```python
from build123d import *

# Parameters (mm, degrees)
F0_W        = 31.6318599507
F0_H        = 42.7960464731
F0_W_2      = 4.3416279368
F0_H_2      = 18.813719973
F0_W_3      = 4.5483717695
F0_H_3      = 19.0204642713
F1_DEPTH    = 3.302
F3_DEPTH    = 0.254
F4_DEPTH    = 12.192
F5_DEPTH    = 7.62
F6_DEPTH    = 7.366
F7_R        = 5.08
F8_T1_DEPTH = 55.4253023246
F9_W        = 5.16293291
F9_H        = 4.0333122015
F9_W_2      = 5.5523253977
F9_H_2      = 4.3130330741
F9_H_3      = 3.302
F9_W_3      = 5.3753489628
F10_DEPTH   = 25.4
F11_R       = 2.4528409794
F12_R       = 1.2264204897


# Not quite as in the source:
# - a fillet or chamfer that OpenCascade refuses, or shapes differently, is made with other operations: its cross-section is extruded or revolved along the edge and cut away or added


with BuildPart() as f1:
    # F0 (on Front) → F1 (new body)
    with BuildSketch(Plane.XZ):
        with Locations((-0.3101159818, 8.9933718555)):
            Rectangle(F0_W, F0_H)
        with Locations((-6.3056976069, 9.4068599865)):
            Rectangle(F0_W_2, F0_H_2, mode=Mode.SUBTRACT)
        with Locations((5.5820937268, 9.5102321357)):
            Rectangle(F0_W_3, F0_H_3, mode=Mode.SUBTRACT)
    extrude(amount=F1_DEPTH)

    # F3 (add): a face of the model
    f3_faces = [f1.faces().sort_by_distance(p)[0] for p in [
        (-0.3101159818, -1.651, 30.391395092),
    ]]
    extrude(f3_faces, amount=F3_DEPTH)

    # F2 (on Top) → F4 (join)
    with BuildSketch(Plane.XY):
        with BuildLine():
            Line((-16.1260459572, -3.0640123878), (-16.1260459572, -5.3753489628))
            Line((-16.1260459572, -5.3753489628), (-16.1260459572, -23.9823255688))
            add(Edge.make_bspline(
                [(-16.1260459572, -23.9823255688), (-10.712885637, -26.1710511495), (-0.0173269949, -30.4956307693), (10.2353861269, -26.1356592233), (15.2990687639, -23.9823255688)],
                knots=[0, 0, 0, 0, 0.5061129111, 1, 1, 1, 1], degree=3))
            Line((15.2990687639, -23.9823255688), (15.2990687639, -5.1686046645))
            Line((15.2990687639, -5.1686046645), (15.2990687639, -3.0640123878))
            Line((15.2990687639, -3.0640123878), (-16.1260459572, -3.0640123878))
        make_face()
    extrude(amount=-F4_DEPTH)

    # F5 (add): a face of the model
    f5_faces = [f1.faces().sort_by_distance(p)[0] for p in [
        (-0.3946759913, -14.5235842944, 0),
    ]]
    extrude(f5_faces, amount=-F5_DEPTH)

    # F6 (add): a face of the model
    f6_faces = [f1.faces().sort_by_distance(p)[0] for p in [
        (-0.3946759913, -14.5235842944, 0),
    ]]
    extrude(f6_faces, amount=-F6_DEPTH)

    # F7
    f7_edges = [f1.edges().sort_by_distance(p)[0] for p in [
        (-0.398964, -28.322485, 0),
        (15.299069, -13.642163, 0),
        (-16.126046, -13.642163, 0),
    ]]
    fillet(f7_edges, radius=F7_R)

    # F8: fillet of radius 5.08 on 1 edges, made by hand

    # F8_s2 → F8_t1 (cut)
    with BuildSketch(Plane.YZ.offset(-28.0227671442)):
        with BuildLine():
            ThreePointArc((-3.302, 25.8867066172), (-2.3956458882, 28.782752197), (0, 30.645395092))
            Line((0, 30.645395092), (-3.302, 30.645395092))
            Line((-3.302, 30.645395092), (-3.302, 25.8867066172))
        make_face()
    extrude(amount=F8_T1_DEPTH, mode=Mode.SUBTRACT)

    # F9 (on face) → F10 (join)
    with BuildSketch(Plane(origin=(0, 0, -12.192), x_dir=(1, 0, 0), z_dir=(0, 0, -1))):
        with Locations((-13.5445795022, 21.965669468)):
            Rectangle(F9_W, F9_H)
        with Locations((12.522906065, 21.8258090317)):
            Rectangle(F9_W_2, F9_H_2)
        with Locations((12.522906065, 1.651)):
            Rectangle(F9_W_2, F9_H_3)
        with Locations((-13.4383714758, 1.651)):
            Rectangle(F9_W_3, F9_H_3)
    extrude(amount=F10_DEPTH)

    # F11
    f11_edges = [f1.edges().sort_by_distance(p)[0] for p in [
        (-8.476512, -3.302, 9.40686),
        (7.85628, -3.302, 9.510232),
        (3.307908, -3.302, 9.510232),
        (-4.134884, -3.302, 9.40686),
    ]]
    fillet(f11_edges, radius=F11_R)

    # F12
    f12_edges = [f1.edges().sort_by_distance(p)[0] for p in [
        (5.582094, -3.302, 19.020464),
        (-6.305698, -3.302, 18.81372),
    ]]
    fillet(f12_edges, radius=F12_R)


solid = f1.part
```
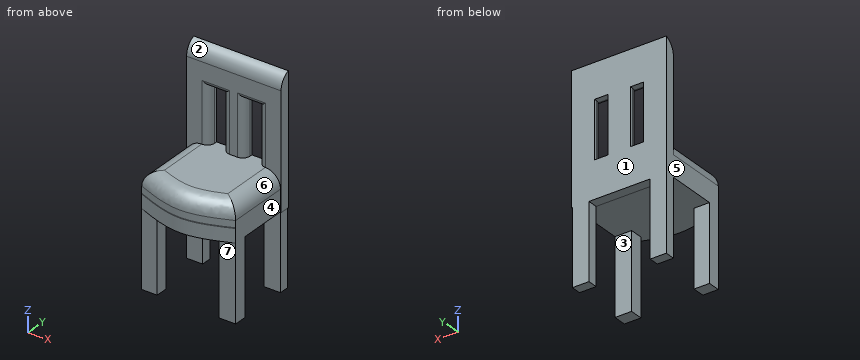
The listing builds one solid part. Answer for the finished solid, in the listing's coordinates (mm). Face numbers are marked on the shaded views. A direction names the side the tool comes from. Coordinates: 2 decimals unless noted, no trailing zeros. Loops run counter-clockwise (first coordinate to the right, second up) from the corner with the lowest first, then second, coordinate; pieces in that order, holes last. Notation, with made-up numbers: (88, 14) -> (116, 14) arc R20 ccw to (116, 23) -> close; hole circle Ø5 at (-21, 40). An arc over 180 degrees is marked (long way). Return JSON: item names as keys, results as strings. Group by question number.
(1) Which of the six approach directions +Z, -Z, +X, -X, +Y, -Y give full straight-line access (tool end or side, diameter ignored) to the marked faces 4, 5, 6 and 7?
(2) A cutting plane is placed at C-C on y = -16.5. Write down the section's boundary in (x, z).
(3) Find the intervals of material crossed by probe 1 along Y at (x, z) = (10.5, -13); probe 2 along Y at (x, z) = (-11, -16.5); probe 3 along X at (y, z) = (-2.75, -34), in increasing order. Write a range as from..to.
(4) Determine the mould class of the marked faces 1, 2 and 3 for opening direction Y: released by +Y, released by -Y, zero draft, split by the parting line, or undercut.
(5) A cutting plane is placed at A-A on z = 16. Write down the section's boundary in (x, y), and give its area (3 significant figures).
(6) A cutting plane is placed at B-B on z = -16.5. Write down the section's boundary in (x, y).
(7) Given pin 1 Ø8 at (x, y) = (2.5, -13.5) entering from +Z; pin 2 Ø8 at (y, z) = (-24, 7.5) entering from -X; pin 3 Ø1 at (y, z) = (-2, -19) entering from +X; pin 4 Ø0.6 at (x, y) = (6.5, -1) entering from -Z, each flat-ended and moving along its own axis, determine where each tip first touches the part or whether it passes through.
The answers:
{
 "1": {"face 4": "+Z, -Z, +X, -Y", "face 5": "+Z, -Z, -X, +Y, -Y", "face 6": "+Z, +X, -Y", "face 7": "-Z, +X, -X, -Y"},
 "2": {"outline": "(-16.13, -12.19) -> (15.3, -12.19) -> (15.3, -5.08) arc R5.08 ccw to (10.22, 0) -> (-11.05, 0) arc R5.08 ccw to (-16.13, -5.08) -> close"},
 "3": {"probe 1": "y = -23.98..-19.67, -3.3..0", "probe 2": "y = -23.98..-19.95, -3.3..0", "probe 3": "x = -16.13..-10.75, 9.75..15.3"},
 "4": {"face 1": "released by +Y", "face 2": "released by -Y", "face 3": "undercut"},
 "5": {"outline": "(-16.13, -3.3) -> (-10.93, -3.3) arc R2.45 ccw to (-8.48, -0.85) -> (-8.48, 0) -> (-16.13, 0) -> close; (-4.13, -0.85) arc R2.45 ccw to (-1.68, -3.3) -> (0.86, -3.3) arc R2.45 ccw to (3.31, -0.85) -> (3.31, 0) -> (-4.13, 0) -> close; (7.86, -0.85) arc R2.45 ccw to (10.31, -3.3) -> (15.51, -3.3) -> (15.51, 0) -> (7.86, 0) -> close", "area": "69.9 mm^2"},
 "6": {"outline": "(-16.13, -23.98) -> (-10.96, -23.98) -> (-10.96, -19.95) -> (-16.13, -19.95) -> close; (-16.13, -3.3) -> (-10.75, -3.3) -> (-10.75, 0) -> (-16.13, 0) -> close; (9.75, -23.98) -> (15.3, -23.98) -> (15.3, -19.67) -> (9.75, -19.67) -> close; (9.75, -3.3) -> (15.3, -3.3) -> (15.3, 0) -> (9.75, 0) -> close"},
 "7": {"pin 1": "stops at z = 0", "pin 2": "passes through", "pin 3": "stops at x = 15.3", "pin 4": "stops at z = -12.4"}
}
